Source: three-view drawing plus pictorial views. Frame: mm from the lowest corner of the part. Round coordinates to 2 decimals unless told otherwise and drop trailing zeros. Loops run counter-clockwise (first coordinate to the right, second up) from the corner with the lowest first, then second, coordinate; pieces in that order, holes last. Notation, with made-up numbers: M 22.5,-12 L 40.5,-12 A15 ccw 40.5,11 Z; hole C 83.5,-24 d1. An arc over 180 degrees is marked long. Return JSON: item names as keys, results as strings. Group by question number.
1) Section C-C (z = 1.1). Output: boundary loops of the cut face in (x, y), plus the area to 3 significant figures.
2) Contact query for flat-ended pins moving along their axis: P1, Ø4, axis at x = 170, y = 5, coming from the +Z side; P2, Ø5.5, axis at x = 23, y = 5, coming from the +Z side. Output: stop coordinate, or through.
3) Material intervals for line 1 (X direction, y = 5, z = 1.75); line 2 (X direction, y = 5, z = 1.05); line 3 (Y direction, x = 96.5, z = 0.65), sorted ascending. Write a range as from..to.
4) Section A-A (y = 5). Count the separate pieces of the cut face and the enclosed holes in it, plus the area to 3 significant figures.
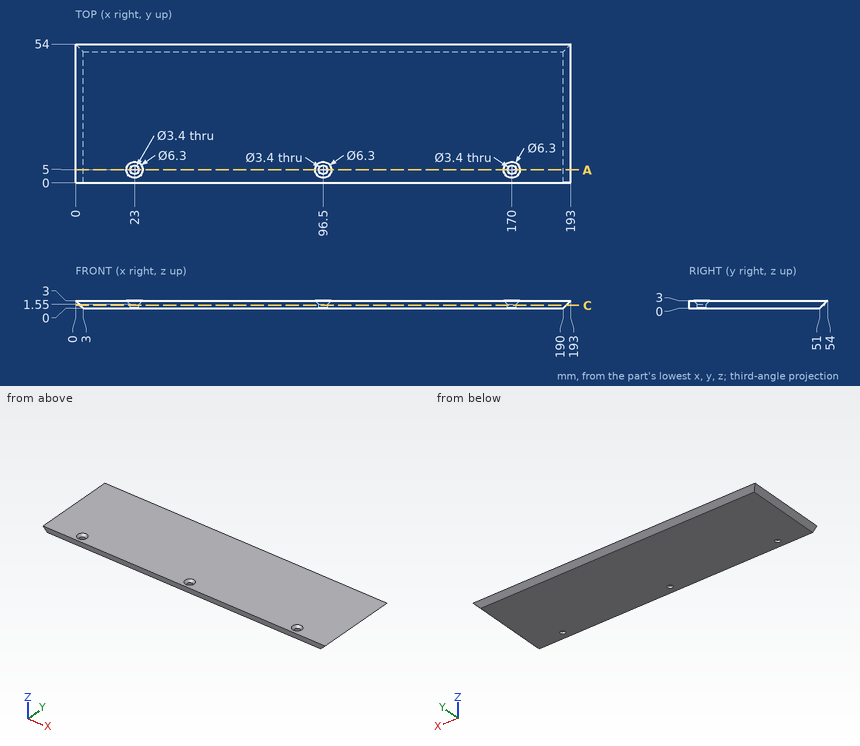
Returned:
{
 "1": {"outline": "M 1.9,0 L 191.1,0 L 191.1,52.1 L 1.9,52.1 Z; hole C 23,5 d3.4; hole C 96.5,5 d3.4; hole C 170,5 d3.4", "area": "9,830 mm^2"},
 "2": {"P1": "stops at z = 1.85", "P2": "stops at z = 2.6"},
 "3": {"line 1": "x = 1.25..21.1, 24.9..94.6, 98.4..168.1, 171.9..191.75", "line 2": "x = 1.95..21.3, 24.7..94.8, 98.2..168.3, 171.7..191.05", "line 3": "y = 0..3.3, 6.7..51.65"},
 "4": {"separate pieces": "4", "enclosed holes": "0", "area": "533 mm^2"}
}
